Verification items for the finished model (mm, model axes). Round coordinates to 2 decimals unless told otherwise and drop trailing zeros. Write each loop counter-clockwise with the first axis right and the second up, starting at its lowest first coordinate (ties: lowest second). Pieces come first, ordered by that corner, then holes. Notation, with made-up numbers: M 61,73.5 L 95,73.5 A14 ccw 95,78.5 Z; hole C -37,-6.5 d2. An arc over 180 degrees is marked long. Write each question's results on one line, items separated by ' | '.
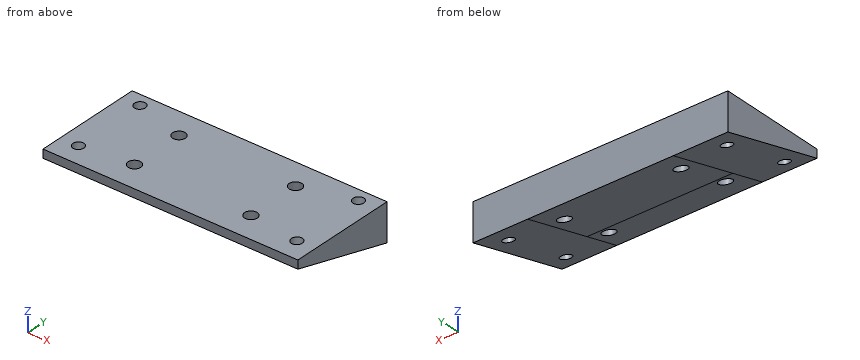
from build123d import *

# Parameters (mm, degrees)
EXTRUDE_1_DEPTH     = 40
EXTRUDE_2_DEPTH     = 40
SKETCH_9_W          = 20.5
SKETCH_9_H          = 20
CUT_EXTRUDE_2_DEPTH = 20
SKETCH_10_W         = 4.875
SKETCH_10_H         = 20
CUT_EXTRUDE_3_DEPTH = 20
CUT_EXTRUDE_4_DEPTH = 55
SKETCH_12_W         = 51.656841865
SKETCH_12_H         = 34.217395835
CUT_EXTRUDE_5_DEPTH = 34
EXTRUDE_3_DEPTH     = 40
SKETCH_16_R         = 1.75
CUT_EXTRUDE_6_DEPTH = 10
EXTRUDE_4_DEPTH     = 15
EXTRUDE_5_DEPTH     = 15
SKETCH_19_R         = 1.5
CUT_EXTRUDE_7_DEPTH = 10


with BuildPart() as part:
    # 草图1 → 凸台-拉伸1 (new body)
    with BuildSketch(Plane.XY):
        Polygon((74.641016151, 0), (74.641016151, 20), (34.641016151, 20), (34.641016151, 9.282032303), (34.641016151, 0), align=None)
    extrude(amount=EXTRUDE_1_DEPTH)

    # 草图8 → 凸台-拉伸2 (add)
    with BuildSketch(Plane(origin=(74.641016151, 0, 0), x_dir=(0, 0, -1), z_dir=(1, 0, 0))):
        Polygon((0, 0), (0, 20), (5.358983849, 20), align=None)
    extrude(amount=-EXTRUDE_2_DEPTH)

    # 草图9 → 切除-拉伸2 (cut)
    with BuildSketch(Plane.XY.offset(40)):
        with Locations((54.641016151, 10)):
            Rectangle(SKETCH_9_W, SKETCH_9_H)
    extrude(amount=-CUT_EXTRUDE_2_DEPTH, mode=Mode.SUBTRACT)

    # 草图10 → 切除-拉伸3 (cut)
    with BuildSketch(Plane.XY.offset(40)):
        with Locations((72.203516151, 10)):
            Rectangle(SKETCH_10_W, SKETCH_10_H)
        with Locations((37.078516151, 10)):
            Rectangle(SKETCH_10_W, SKETCH_10_H)
    extrude(amount=-CUT_EXTRUDE_3_DEPTH, mode=Mode.SUBTRACT)

    # 草图11 → 切除-拉伸4 (cut)
    with BuildSketch(Plane(origin=(74.641016151, 0, 0), x_dir=(0, 0, -1), z_dir=(1, 0, 0))):
        Polygon((0, 0), (5.358983849, 20), (-9.641016151, 20), (-15, 0), align=None)
    extrude(amount=-CUT_EXTRUDE_4_DEPTH, mode=Mode.SUBTRACT)

    # 草图12 → 切除-拉伸5 (cut)
    with BuildSketch(Plane.XY.offset(20)):
        with Locations((55.994076619, 8.947658785)):
            Rectangle(SKETCH_12_W, SKETCH_12_H)
    extrude(amount=CUT_EXTRUDE_5_DEPTH, mode=Mode.SUBTRACT)

    # 草图15 → 凸台-拉伸3 (add)
    with BuildSketch(Plane.ZY.offset(-34.641016151)):
        Polygon((20, 0), (20, -10), (17.679491924, -10), (15, 0), align=None)
    extrude(amount=-EXTRUDE_3_DEPTH)

    # 草图16 → 切除-拉伸6 (cut)
    with BuildSketch(Plane.XY.offset(20)):
        with Locations((38.641016151, 12.5)):
            Circle(SKETCH_16_R)
        with Locations((70.641016151, 12.5)):
            Circle(SKETCH_16_R)
        with Locations((70.641016151, -2.5)):
            Circle(SKETCH_16_R)
        with Locations((38.641016151, -2.5)):
            Circle(SKETCH_16_R)
    extrude(amount=-CUT_EXTRUDE_6_DEPTH, mode=Mode.SUBTRACT)

    # 草图17 → 凸台-拉伸4 (add)
    with BuildSketch(Plane(origin=(74.641016151, 0, 0), x_dir=(0, 0, -1), z_dir=(1, 0, 0))):
        Polygon((-20, 20), (-20, -10), (-17.679491924, -10), (-9.641016151, 20), align=None)
    extrude(amount=EXTRUDE_4_DEPTH)

    # 草图18 → 凸台-拉伸5 (add)
    with BuildSketch(Plane.ZY.offset(-34.641016151)):
        Polygon((20, 20), (9.641016151, 20), (17.679491924, -10), (20, -10), align=None)
    extrude(amount=EXTRUDE_5_DEPTH)

    # 草图19 → 切除-拉伸7 (cut)
    with BuildSketch(Plane(origin=(0, 3.75, 13.995190528), x_dir=(-1, 0, 0), z_dir=(0, -0.2588190451025213, -0.9659258262890682))):
        with Locations(Location((-84.641016151, -9.235047481, 0), (0, 0, 90))):
            Circle(SKETCH_19_R)
        with Locations(Location((-84.641016151, 10.764952519, 0), (0, 0, 90))):
            Circle(SKETCH_19_R)
        with Locations(Location((-24.641016151, -9.235047481, 0), (0, 0, 90))):
            Circle(SKETCH_19_R)
        with Locations(Location((-24.641016151, 10.764952519, 0), (0, 0, 90))):
            Circle(SKETCH_19_R)
    extrude(amount=-CUT_EXTRUDE_7_DEPTH, mode=Mode.SUBTRACT)


solid = part.part
1) Depth check by flat-ended pin: P1, Ø4, axis at x = 38.64, y = 12.5, coming from the -Z side; P2, Ø5.5, axis at x = 70.64, y = 12.5, coming from the +Z side. Enter the tip coordinate at first touch or a pass-through.
Calculated:
P1: stops at z = 11.11 | P2: stops at z = 20
2) Sectioned sample at C-C, the plane x = 51.5. Record the cut outline in (y, z), and give its area (3 significant figures).
Calculated:
outline: M -10,17.68 L 20,9.64 L 20,20 L -10,20 Z | area: 190 mm²
3) Sectioned sample at D-D, the plane y = 5.5. Record the cut outline in (x, z), and give its area (3 significant figures).
Calculated:
outline: M 19.64,13.53 L 89.64,13.53 L 89.64,20 L 19.64,20 Z | area: 453 mm²
4) Sectioned sample at B-B, the plane x = 84. Record the cut outline in (y, z), and give its area (3 significant figures).
Calculated:
outline: M -10,17.68 L -6.48,16.74 L -5.61,20 L -10,20 Z; M -3.86,16.03 L 12.84,11.56 L 15.1,20 L -2.8,20 Z; M 15.46,10.86 L 20,9.64 L 20,20 L 17.91,20 Z | area: 155 mm²
5) Sectioned sample at A-A, the plane y = 11.5. Record the cut outline in (x, z), and give its area (3 significant figures).
Calculated:
outline: M 19.64,11.92 L 37.2,11.92 L 37.2,20 L 19.64,20 Z; M 40.08,11.92 L 69.2,11.92 L 69.2,20 L 40.08,20 Z; M 72.08,11.92 L 89.64,11.92 L 89.64,20 L 72.08,20 Z | area: 519 mm²
6) Material ranges on line 1 (X direction, y = -2.5, z = 18.65); line 2 (X direction, y = 13, z = 16.5); line 3 (Z direction, x = 71.5, y = -0.75), recorded low to high. Write a range as [from, to].
Calculated:
line 1: x = [19.64, 36.89], [40.39, 68.89], [72.39, 89.64] | line 2: x = [19.64, 36.96], [40.32, 68.96], [72.32, 89.64] | line 3: z = [15.2, 20]
